Could you check a few things on this drawing? It's one solid part, dimensions in mm from its lowest x, y, z. A direction names the side the tool comes from. Round coordinates to 2 decimals unless told otherwise and drop trailing zeros. Order: outer loops, then holes, each group sorted by start corner. A loop starts at its lowest first (then second) coordinate and runs counter-clockwise, first axis right, second up. Notation, with made-up numbers: (67, -5.5) -> (77, -5.5) arc R21 ccw to (77, 33.5) -> close; hole circle Ø5 at (50, 2). An arc over 180 degrees is marked (long way). Use a Markdown table: item, result. Add a question column.
(1) I want a section at C-C, the plane x = 107. Please give me the cut outline in (y, z).
(2) I want a section at B-B, the plane y = 38.5. Please give me the cut outline in (x, z).
(3) On a 3-axis mill with a long thin cutter (end or side, diameter ignored), from which of +Z, -Z, +X, -X, +Y, -Y can I reach the whole of each face in a straight line? I mean the marked faces 4, 5, 6 and 7. Say none if no direction works.
(4) Thinking about a two-plate mould opening in Z: for the marked faces 1, 2 and 3, which applies, pulls with the +Z half, pulls with the -Z half, needs draft (parallel to the pull), parting line crosses it, or undercut?
(5) I want a section at D-D, the plane y = 62. Please give me the cut outline in (x, z), then the cut area to 3 significant figures.
(6) If I drill on probe 1 along X at (y, z) = (18, 50); probe 2 along X at (y, z) = (37, 50.8); probe 3 along X at (y, z) = (33.5, 4.5), over which ranges is the centre line in solid material (lowest first)?
(7) I want a section at A-A, the plane z = 9. Please give me the cut outline in (x, y), then the cut area to 3 significant figures.
(8) I'm going to push a flat-ended pin straight in: P1, Ø7.5, axis at y = 13.5, z = 58, coming from the -X side. Where does the tip first touch, or does it pass through?
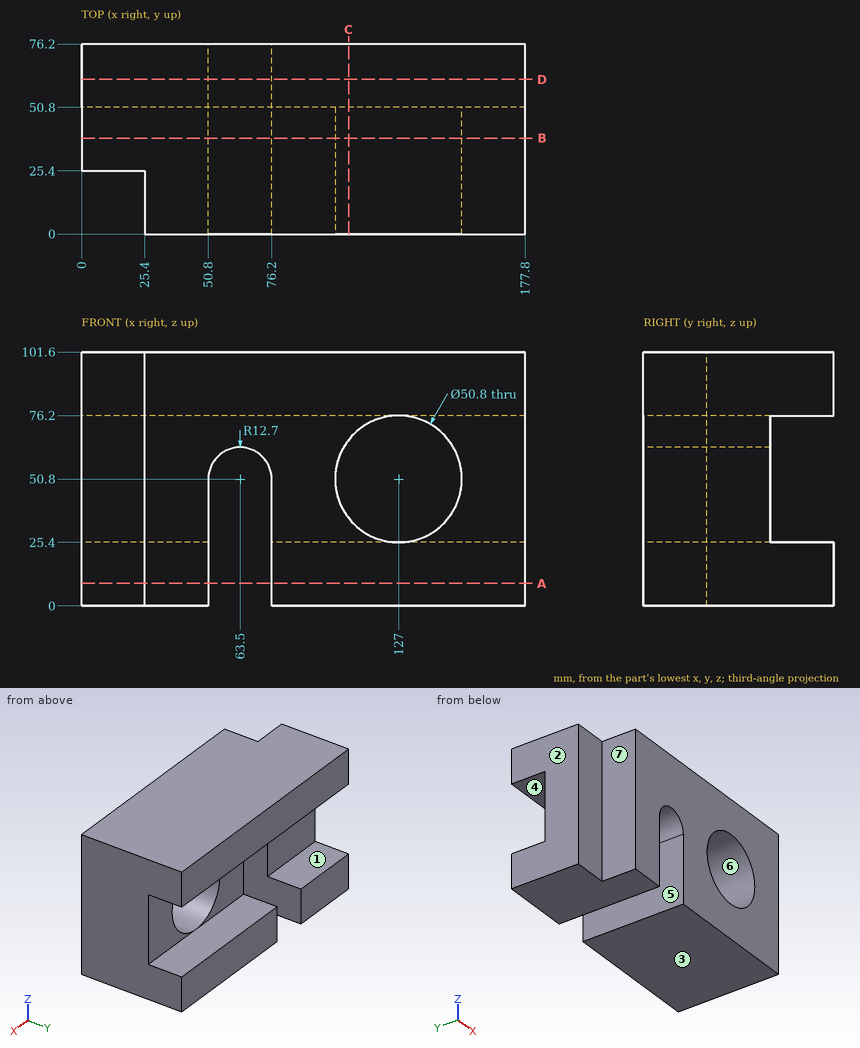
Taken from the geometry:
| question | item | result |
|---|---|---|
| 1 | outline | (0, 0) -> (76.2, 0) -> (76.2, 25.4) -> (50.8, 25.4) -> (50.8, 35.14) -> (0, 35.14) -> close; (0, 66.46) -> (50.8, 66.46) -> (50.8, 76.2) -> (76.2, 76.2) -> (76.2, 101.6) -> (0, 101.6) -> close |
| 2 | outline | (0, 0) -> (50.8, 0) -> (50.8, 50.8) arc R12.7 cw to (76.2, 50.8) -> (76.2, 0) -> (177.8, 0) -> (177.8, 101.6) -> (0, 101.6) -> close; hole circle Ø50.8 at (127, 50.8) |
| 3 | face 4 | +X, -X, +Y |
| 3 | face 5 | -Z, +Y, -Y |
| 3 | face 6 | +Y, -Y |
| 3 | face 7 | +Z, -Z, -X, -Y |
| 4 | face 1 | undercut |
| 4 | face 2 | needs draft |
| 4 | face 3 | pulls with the -Z half |
| 5 | outline | (0, 0) -> (50.8, 0) -> (50.8, 25.4) -> (0, 25.4) -> close; (0, 76.2) -> (177.8, 76.2) -> (177.8, 101.6) -> (0, 101.6) -> close; (76.2, 0) -> (177.8, 0) -> (177.8, 25.4) -> (76.2, 25.4) -> close |
| 5 | area | 8,390 mm2 |
| 6 | probe 1 | x = 25.4 to 50.8, 76.2 to 101.61, 152.39 to 177.8 |
| 6 | probe 2 | x = 0 to 50.8, 76.2 to 101.6, 152.4 to 177.8 |
| 6 | probe 3 | x = 0 to 50.8, 76.2 to 177.8 |
| 7 | outline | (0, 25.4) -> (25.4, 25.4) -> (25.4, 0) -> (50.8, 0) -> (50.8, 76.2) -> (0, 76.2) -> close; (76.2, 0) -> (177.8, 0) -> (177.8, 76.2) -> (76.2, 76.2) -> close |
| 7 | area | 11,000 mm2 |
| 8 | P1 | stops at x = 25.4 |
